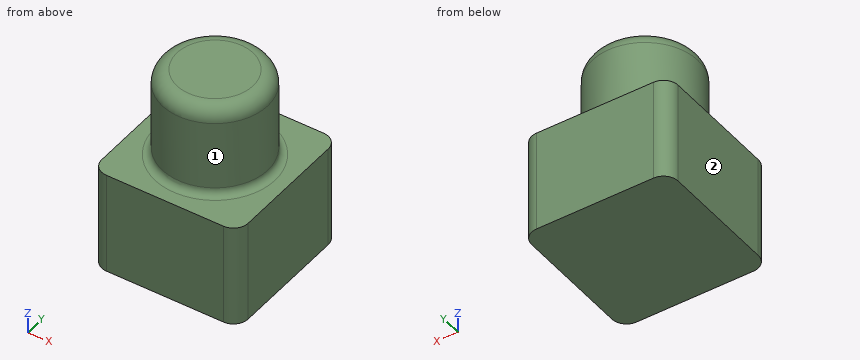
```python
from build123d import *

# Parameters (mm, degrees)
CYLINDER_R     = 3.6
CYLINDER_DEPTH = 6.2
BOX_W          = 10
BOX_H          = 10
BOX_DEPTH      = 7
FILLET_R       = 1
FILLET001_R    = 0.5
FILLET002_R    = 1


with BuildPart() as cylinder:
    # Cylinder → Cylinder (new body)
    with BuildSketch(Plane.XY):
        Circle(CYLINDER_R)
    extrude(amount=CYLINDER_DEPTH)


with BuildPart() as fillet002:
    # Box → Box (new body)
    with BuildSketch(Plane(origin=(-5, -5, -7), x_dir=(1, 0, 0), z_dir=(0, 0, 1))):
        with Locations((5, 5)):
            Rectangle(BOX_W, BOX_H)
    extrude(amount=BOX_DEPTH)

    # Fusion: union Cylinder
    add(cylinder.part)

    # Fillet
    fillet_edges = [fillet002.edges().sort_by_distance(p)[0] for p in [
        (-5, -5, -3.5),
        (-5, 5, -3.5),
        (5, -5, -3.5),
        (5, 5, -3.5),
    ]]
    fillet(fillet_edges, radius=FILLET_R)

    # Fillet001
    fillet001_edges = [fillet002.edges().sort_by_distance(p)[0] for p in [
        (-3.6, 0, 0),
    ]]
    fillet(fillet001_edges, radius=FILLET001_R)

    # Fillet002
    fillet002_edges = [fillet002.edges().sort_by_distance(p)[0] for p in [
        (-3.6, 0, 6.2),
    ]]
    fillet(fillet002_edges, radius=FILLET002_R)


solid = fillet002.part
```
Here's how the part is built. I have some questions about the finished solid (model axes, mm). Face numbers are marked on the shaded views. A direction names the side the tool comes from. Give positions to 0.01 mm unless a question says otherwise; leave off trailing zeros. Loops run counter-clockwise (first coordinate to the right, second up) from the corner with the lowest first, then second, coordinate; pieces in that order, holes last. Notation, with made-up numbers: M 76.5,8 L 125.5,8 A18 ccw 125.5,27 Z; hole C -6,35 d10. An arc over 180 degrees is marked long. Return JSON: item names as keys, results as strings.
Item 1: I'm going to push flat-ended pins straight in: pin 1 Ø4 at (x, z) = (2.5, 3) entering from -Y; pin 2 Ø1 at (y, z) = (-0.5, 3.5) entering from +X. Where does each tip first touch, or does it pass through?
A:
{"pin 1": "stops at y = -3.57", "pin 2": "stops at x = 3.6"}
Item 2: Imagine slicing it at A-A on y = 0. List the corners of the cut face in (x, z) for me.
A:
{"outline": "M -5,-7 L 5,-7 L 5,0 L 4.1,0 A0.5 cw 3.6,0.5 L 3.6,5.2 A1 ccw 2.6,6.2 L -2.6,6.2 A1 ccw -3.6,5.2 L -3.6,0.5 A0.5 cw -4.1,0 L -5,0 Z"}
Item 3: Imagine slicing it at C-C on z = 1.25. List the corners of the cut face in (x, y) for me.
A:
{"outline": "C 0,0 d7.2"}
Item 4: Please list where these lines run through material, in increasing order: line 1 (Z direction, x = 4.25, y = 3.5); line 2 (Z direction, x = 3.5, y = 0.25); line 3 (X direction, y = -4.25, z = -0.5).
A:
{"line 1": "z = -7 to 0", "line 2": "z = -7 to 5.62", "line 3": "x = -4.97 to 4.97"}
Item 5: On a 3-axis mill with a long thin cutter (end or side, diameter ignored), from which of +Z, -Z, +X, -X, +Y, -Y can I reach the whole of each face in a straight line? I mean the marked faces 1 and 2. Say none if no direction works.
A:
{"face 1": "+Z", "face 2": "+Z, -Z, -X, +Y, -Y"}
